Check sheet for the modelled part. Datum: model origin and axes. Units: mm. Give positions to 0.01 mm unless a question says otherwise; leave off trailing zeros. Write each loop counter-clockwise with the first axis right and the second up, starting at its lowest first coordinate (ties: lowest second). Pieces come first, ordered by that corner, then holes. Notation, with made-up numbers: (64, 9) -> (85, 9) arc R32 ccw to (85, 42) -> close; hole circle Ø10 at (26.25, 88.5). An arc over 180 degrees is marked (long way). Write each question's results on one line, items separated by ' | '. Start each with the question number.
```python
from build123d import *

# Parameters (mm, degrees)
CROQUIS1_W                                      = 497.15
CROQUIS1_H                                      = 80
BRIDA_BASE1_DEPTH                               = 6.35
REDONDEO1_R                                     = 2
TALADRO_DE_MARGEN_PARA_M51_D                    = 5.5
CORTAR_EXTRUIR1_DEPTH                           = 10
CROQUIS10_R                                     = 3
CORTAR_EXTRUIR2_DEPTH                           = 10
SKETCH1_R                                       = 4.5
CUT_EXTRUDE1_DEPTH                              = 6.35
CSK_FOR_M8_OVAL_HEAD_MACHINE_SCREW1_D           = 9
CSK_FOR_M8_OVAL_HEAD_MACHINE_SCREW1_DEPTH       = 6.349
CSK_FOR_M8_OVAL_HEAD_MACHINE_SCREW1_CSINK_D     = 17.3
CSK_FOR_M8_OVAL_HEAD_MACHINE_SCREW1_CSINK_ANGLE = 90
CSK_FOR_M8_OVAL_HEAD_MACHINE_SCREW1_TIP         = 2.703872786


# Sheet-metal steps are written as plain solids
with BuildPart() as part:
    # Croquis1 → Brida base1 (new body)
    with BuildSketch(Plane(origin=(0, 0, 0), x_dir=(1, 0, 0), z_dir=(0, 1, 0))):
        with Locations((98.797222222, -5.555555556)):
            Rectangle(CROQUIS1_W, CROQUIS1_H)
    extrude(amount=-BRIDA_BASE1_DEPTH)

    # Redondeo1
    redondeo1_edges = [part.edges().sort_by_distance(p)[0] for p in [
        (-149.777777778, -3.175, -34.444444444),
        (-149.777777778, -3.175, 45.555555556),
    ]]
    fillet(redondeo1_edges, radius=REDONDEO1_R)

    # Taladro de margen para M51 (through all)
    with Locations(Plane(origin=(0, 0, 0), x_dir=(1, 0, 0), z_dir=(0, 1, 0))):
        with Locations((-119.777777778, 24.444444444), (-119.777777778, -35.555555556), (80.222222222, -35.555555556), (80.222222222, 24.444444444)):
            Hole(TALADRO_DE_MARGEN_PARA_M51_D / 2)

    # Croquis9 → Cortar-Extruir1 (cut)
    with BuildSketch(Plane(origin=(0, -6.35, 0), x_dir=(-1, 0, 0), z_dir=(0, -1, 0))):
        with BuildLine():
            Line((-307.372222222, 14.444444444), (-277.234752083, 14.444444444))
            ThreePointArc((-277.234752083, 14.444444444), (-257.234752083, -5.555555556), (-277.234752083, -25.555555556))
            Line((-277.234752083, -25.555555556), (-307.372222222, -25.555555556))
            ThreePointArc((-307.372222222, -25.555555556), (-327.372222222, -5.555555556), (-307.372222222, 14.444444444))
        make_face()
        with BuildLine():
            Line((-50.222222222, 14.444444444), (99.777777778, 14.444444444))
            ThreePointArc((99.777777778, 14.444444444), (119.777777778, -5.555555556), (99.777777778, -25.555555556))
            Line((99.777777778, -25.555555556), (-50.222222222, -25.555555556))
            ThreePointArc((-50.222222222, -25.555555556), (-70.222222222, -5.555555556), (-50.222222222, 14.444444444))
        make_face()
        with BuildLine():
            Line((-214.481912447, 14.444444444), (-110.222222222, 14.444444444))
            ThreePointArc((-110.222222222, 14.444444444), (-90.222222222, -5.555555556), (-110.222222222, -25.555555556))
            Line((-110.222222222, -25.555555556), (-214.481912447, -25.555555556))
            ThreePointArc((-214.481912447, -25.555555556), (-234.481912447, -5.555555556), (-214.481912447, 14.444444444))
        make_face()
    extrude(amount=-CORTAR_EXTRUIR1_DEPTH, mode=Mode.SUBTRACT)

    # Croquis10 → Cortar-Extruir2 (cut)
    with BuildSketch(Plane.XZ.offset(6.35)):
        with Locations(Location((332.372222222, 17.555555556, 0), (0, 0, 270))):
            Circle(CROQUIS10_R)
        with Locations(Location((246.372222222, 17.555555556, 0), (0, 0, 270))):
            Circle(CROQUIS10_R)
        with Locations(Location((246.372222222, -6.444444444, 0), (0, 0, 270))):
            Circle(CROQUIS10_R)
        with Locations(Location((332.372222222, -6.444444444, 0), (0, 0, 270))):
            Circle(CROQUIS10_R)
    extrude(amount=-CORTAR_EXTRUIR2_DEPTH, mode=Mode.SUBTRACT)

    # Sketch1 → Cut-Extrude1 (cut)
    with BuildSketch(Plane.XZ.offset(6.35)):
        with Locations(Location((-44.777777778, -24.444444444, 0), (0, 0, 270))):
            Circle(SKETCH1_R)
        with Locations(Location((5.222222222, -24.444444444, 0), (0, 0, 270))):
            Circle(SKETCH1_R)
        with Locations(Location((5.222222222, 35.555555556, 0), (0, 0, 270))):
            Circle(SKETCH1_R)
        with Locations(Location((-44.777777778, 35.555555556, 0), (0, 0, 90))):
            Circle(SKETCH1_R)
    extrude(amount=-CUT_EXTRUDE1_DEPTH, mode=Mode.SUBTRACT)

    # CSK for M8 Oval Head Machine Screw1
    with Locations(Plane(origin=(5.222222222, -6.35, 35.555555556), x_dir=(0, 0, -1), z_dir=(0, -1, 0))):
        with Locations((0, 0), (0, -50), (60, -50), (60, 0)):
            CounterSinkHole(CSK_FOR_M8_OVAL_HEAD_MACHINE_SCREW1_D / 2, CSK_FOR_M8_OVAL_HEAD_MACHINE_SCREW1_CSINK_D / 2, depth=CSK_FOR_M8_OVAL_HEAD_MACHINE_SCREW1_DEPTH, counter_sink_angle=CSK_FOR_M8_OVAL_HEAD_MACHINE_SCREW1_CSINK_ANGLE)
            with Locations((0, 0, -(CSK_FOR_M8_OVAL_HEAD_MACHINE_SCREW1_DEPTH + CSK_FOR_M8_OVAL_HEAD_MACHINE_SCREW1_TIP / 2))):  # 118° drill point
                Cone(0, CSK_FOR_M8_OVAL_HEAD_MACHINE_SCREW1_D / 2, CSK_FOR_M8_OVAL_HEAD_MACHINE_SCREW1_TIP, mode=Mode.SUBTRACT)


solid = part.part
```
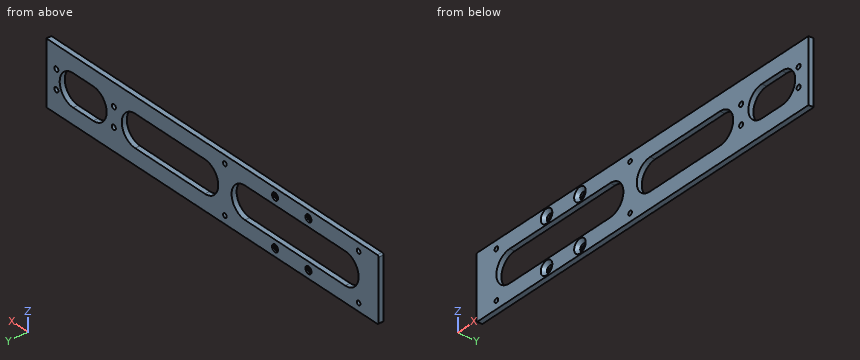
Item 1: Depth check by flat-ended pin: pin 1 Ø9 at (x, z) = (80.22, -24.44) entering from -Y. Enter the tip coordinate at first touch or a pass-through.
Item 2: Section check A-A on x = 283. Record the boundary of the cut face in (y, z).
Item 3: Section check C-C on z = 9. Record the boundary of the cut face in (x, y).
Item 4: Section check B-B on y = -4. Count the separate pieces of the cut face and the enclosed holes in it, then the cut area to 3 significant figures.
Item 5: Thickness scan on probe 1 along Z at (x, y) = (-69, -2.75); probe 2 along X at (y, z) = (-4.25, -9); probe 3 along X at (y, z) = (-1, -23). Record the ranges inside material, lowest first. Write a range as from..to.
Check sheet entries:
1) pin 1: stops at y = -6.35
2) outline: (-6.35, -34.44) -> (0, -34.44) -> (0, -14.44) -> (-6.35, -14.44) -> close; (-6.35, 25.56) -> (0, 25.56) -> (0, 45.56) -> (-6.35, 45.56) -> close
3) outline: (-149.78, -6.35) -> (-119.48, -6.35) -> (-119.48, 0) -> (-149.78, 0) -> close; (69.92, -6.35) -> (90.52, -6.35) -> (90.52, 0) -> (69.92, 0) -> close; (234.18, -6.35) -> (257.53, -6.35) -> (257.53, 0) -> (234.18, 0) -> close; (327.07, -6.35) -> (347.37, -6.35) -> (347.37, 0) -> (327.07, 0) -> close
4) separate pieces: 1 | enclosed holes: 15 | area: 23,900 mm^2
5) probe 1: z = -34.44..-14.44, 25.56..45.56 | probe 2: x = -149.78..-113.49, 63.94..96.51, 228.2..244.8, 247.94..263.52, 321.09..330.8, 333.94..347.37 | probe 3: x = -149.78..-122.12, -117.44..-49.04, -40.52..0.96, 9.48..77.88, 82.56..347.37
